Verification items for the finished model (mm, model axes). Round coordinates to 2 decimals unless told otherwise and drop trailing zeros. Loops run counter-clockwise (first coordinate to the right, second up) from the corner with the lowest first, then second, coordinate; pieces in that order, holes last. Notation, with made-up numbers: (-38, 13.25) -> (-25, 13.25) arc R25 cw to (-25, 27.25) -> close; hole circle Ø11 at (24, 66.5). An arc over 180 degrees is marked (long way). Write item = value, one per line. Start each with the question number.
```python
from build123d import *

# Parameters (mm, degrees)
SKETCH2_R = 0.75


with BuildPart() as part:
    # Sweep1: sweep along a path in Sketch1
    with BuildLine(Plane(origin=(0, 0, 0), x_dir=(1, 0, 0), z_dir=(0, 1, 0))) as sweep1_path:
        Line((-0.5, -7.5), (0.5, -7.5))
        ThreePointArc((0.5, -7.5), (5.449747468, -5.449747468), (7.5, -0.5))
        Line((7.5, -0.5), (7.5, 0.5))
        ThreePointArc((7.5, 0.5), (5.449747468, 5.449747468), (0.5, 7.5))
        Line((0.5, 7.5), (-0.5, 7.5))
        ThreePointArc((-0.5, 7.5), (-5.449747468, 5.449747468), (-7.5, 0.5))
        Line((-7.5, 0.5), (-7.5, -0.5))
        ThreePointArc((-7.5, -0.5), (-5.449747468, -5.449747468), (-0.5, -7.5))
    # Sketch2 → Sweep1 (sweep)
    with BuildSketch(Plane(origin=(0, 0, 0), x_dir=(0, 0, -1), z_dir=(1, 0, 0))):
        with Locations((7.5, 0)):
            Circle(SKETCH2_R)
    sweep(path=sweep1_path.line)


solid = part.part
```
(1) Draft check along Z on faces 1 (the cylindrical face through (-6.75, -0.03, 0.01)), 2 (the cylindrical face through (-0.01, -0.03, -6.75)). Enter one of: +Z half, -Z half, draft (parallel to the pull), parting line (faces both ways), or undercut.
(2) Scan lines: line 1 (X direction, y = -0.05, z = -5.5); line 2 (X direction, y = -0.6, z = -5.5); line 3 (Z direction, x = -4.25, y = -0.25). Record each from-to range of solid material in increasing order. Write a range as [from, to].
(3) Section check A-A on y = 0. Enter the section's corners in (x, z), then the cut area to 3 significant figures.
Computed values:
q1.face_1 = undercut
q1.face_2 = undercut
q2.line_1 = [-6.42, -4.25], [4.25, 6.42]
q2.line_2 = [-6.02, -4.73], [4.73, 6.02]
q2.line_3 = [-7.23, -5.55], [5.55, 7.23]
q3.outline = (-8.25, -0.5) arc R7.75 ccw to (-0.5, -8.25) -> (0.5, -8.25) arc R7.75 ccw to (8.25, -0.5) -> (8.25, 0.5) arc R7.75 ccw to (0.5, 8.25) -> (-0.5, 8.25) arc R7.75 ccw to (-8.25, 0.5) -> close; hole (-6.75, -0.5) arc R6.25 ccw to (-0.5, -6.75) -> (0.5, -6.75) arc R6.25 ccw to (6.75, -0.5) -> (6.75, 0.5) arc R6.25 ccw to (0.5, 6.75) -> (-0.5, 6.75) arc R6.25 ccw to (-6.75, 0.5) -> close
q3.area = 72.0 mm²
